from build123d import *

# Parameters (mm, degrees)
SKETCH_1_R          = 19
SKETCH_1_R_2        = 1.45
SKETCH_1_R_3        = 2
EXTRUDE_1_DEPTH     = 12
SKETCH_2_R          = 1.45
SKETCH_2_R_2        = 2
EXTRUDE_2_DEPTH     = 7
SKETCH_3_R          = 1.45
CUT_EXTRUDE_1_DEPTH = 50.298411063
SKETCH_4_R          = 1.45
CUT_EXTRUDE_2_DEPTH = 50.298411063
SKETCH_5_R          = 1.45
CUT_EXTRUDE_3_DEPTH = 8
SKETCH_6_R          = 1.45
CUT_EXTRUDE_4_DEPTH = 46.489925625
CHAMFER_1_SIZE      = 1.55


with BuildPart() as part:
    # 草图1 → 凸台-拉伸1 (new body)
    with BuildSketch(Plane(origin=(0, 0, 0), x_dir=(1, 0, 0), z_dir=(0, 1, 0))):
        with Locations(Location((0, 0, 0), (0, 0, 270))):
            Circle(SKETCH_1_R)
        with Locations(Location((0, 13.5, 0), (0, 0, 270))):
            Circle(SKETCH_1_R_2, mode=Mode.SUBTRACT)
        with Locations(Location((-11.691342951, -6.75, 0), (0, 0, 270))):
            Circle(SKETCH_1_R_2, mode=Mode.SUBTRACT)
        with Locations(Location((11.691342951, -6.75, 0), (0, 0, 270))):
            Circle(SKETCH_1_R_2, mode=Mode.SUBTRACT)
        with Locations(Location((-10.522208656, 6.075, 0), (0, 0, 270))):
            Circle(SKETCH_1_R_3, mode=Mode.SUBTRACT)
        with Locations(Location((0, -12.15, 0), (0, 0, 270))):
            Circle(SKETCH_1_R_3, mode=Mode.SUBTRACT)
        with Locations(Location((10.522208656, 6.075, 0), (0, 0, 270))):
            Circle(SKETCH_1_R_3, mode=Mode.SUBTRACT)
    extrude(amount=EXTRUDE_1_DEPTH)

    # 草图2 → 凸台-拉伸2 (add)
    with BuildSketch(Plane(origin=(0, 12, 0), x_dir=(1, 0, 0), z_dir=(0, 1, 0))):
        Polygon((0, 21.939310229), (-19, 10.969655115), (-19, -10.969655115), (0, -21.939310229), (19, -10.969655115), (19, 10.969655115), align=None)
        with Locations(Location((0, 13.5, 0), (0, 0, 270))):
            Circle(SKETCH_2_R, mode=Mode.SUBTRACT)
        with Locations(Location((-10.522208656, 6.075, 0), (0, 0, 270))):
            Circle(SKETCH_2_R_2, mode=Mode.SUBTRACT)
        with Locations(Location((10.522208656, 6.075, 0), (0, 0, 270))):
            Circle(SKETCH_2_R_2, mode=Mode.SUBTRACT)
        with Locations(Location((-11.691342951, -6.75, 0), (0, 0, 270))):
            Circle(SKETCH_2_R, mode=Mode.SUBTRACT)
        with Locations(Location((0, -12.15, 0), (0, 0, 270))):
            Circle(SKETCH_2_R_2, mode=Mode.SUBTRACT)
        with Locations(Location((11.691342951, -6.75, 0), (0, 0, 270))):
            Circle(SKETCH_2_R, mode=Mode.SUBTRACT)
    extrude(amount=-EXTRUDE_2_DEPTH)

    # 草图3 → 切除-拉伸1 (cut, through all)
    with BuildSketch(Plane(origin=(9.5, 0, 16.454482672), x_dir=(0.8660254037844384, 0, -0.5000000000000004), z_dir=(0.5000000000000004, 0, 0.8660254037844384))):
        with Locations((0, 8.5)):
            Circle(SKETCH_3_R)
    extrude(amount=-CUT_EXTRUDE_1_DEPTH, mode=Mode.SUBTRACT)

    # 草图4 → 切除-拉伸2 (cut, through all)
    with BuildSketch(Plane(origin=(-9.5, 0, 16.454482672), x_dir=(0.8660254037844385, 0, 0.5000000000000004), z_dir=(-0.5000000000000003, 0, 0.8660254037844384))):
        with Locations((0, 8.5)):
            Circle(SKETCH_4_R)
    extrude(amount=-CUT_EXTRUDE_2_DEPTH, mode=Mode.SUBTRACT)

    # 草图5 → 切除-拉伸3 (cut)
    with BuildSketch(Plane.ZY.offset(19)):
        with Locations((0, 8.5)):
            Circle(SKETCH_5_R)
    extrude(amount=-CUT_EXTRUDE_3_DEPTH, mode=Mode.SUBTRACT)

    # 草图6 → 切除-拉伸4 (cut, through all)
    with BuildSketch(Plane(origin=(19, 0, 0), x_dir=(0, 0, -1), z_dir=(1, 0, 0))):
        with Locations(Location((0, 8.5, 0), (0, 0, 180))):
            Circle(SKETCH_6_R)
    extrude(amount=-CUT_EXTRUDE_4_DEPTH, mode=Mode.SUBTRACT)

    # 倒角1
    chamfer_1_edges = [part.edges().sort_by_distance(p)[0] for p in [
        (11.691342951, 12, 5.3),
        (0, 12, -14.95),
        (-11.691342951, 12, 5.3),
    ]]
    chamfer(chamfer_1_edges, length=CHAMFER_1_SIZE)


solid = part.part
Verification items for the finished model (mm, model axes). A direction names the side the tool comes from. Give positions to 0.01 mm unless a question says otherwise; leave off trailing zeros. Write each loop counter-clockwise with the first axis right and the second up, starting at its lowest first coordinate (ties: lowest second). Pieces come first, ordered by that corner, then holes. Notation, with made-up numbers: M 24.5,81 L 30.5,81 A18 cw 30.5,103 Z; hole C 82,-9.5 d6. An arc over 180 degrees is marked long. Write item = value, one per line.
(1) Material ranges on line 1 (Y direction, x = -11, z = 0); line 2 (X direction, y = 8, z = 6.75); line 3 (Z direction, x = -0.5, y = 10.5), recorded low to high.
Found:
line_1 = 0 to 7.05, 9.95 to 12
line_2 = -19 to -13.14, -10.24 to -5.47, -2.33 to 2.33, 5.47 to 10.24, 13.14 to 19
line_3 = -21.65 to -14.91, -12.09 to 10.21, 14.09 to 21.65
(2) Sectioned sample at C-C (y = 6). Record the cut outline in (x, z) (3 decimals).
Found:
outline = M -19,-10.97 L 0,-21.939 L 19,-10.97 L 19,10.97 L 0,21.939 L -19,10.97 Z; hole C -11.691,6.75 d2.9; hole C -10.522,-6.075 d4; hole C 0,12.15 d4; hole C 0,-13.5 d2.9; hole C 10.522,-6.075 d4; hole C 11.691,6.75 d2.9
(3) Sectioned sample at B-B (z = 18). Record the cut outline in (x, y).
Found:
outline = M -6.82,5 L -6.08,5 L -6.08,0 L 6.08,0 L 6.08,5 L 6.82,5 L 6.82,12 L -6.82,12 Z
(4) Access from +Z, -Z, +X, -X, +Y, -Y to the whole of each face (thin tool, end or side, straight path). Record for faces 1 (the face through (-5.94, 8.56, -7.39)), 2 (the face through (17, 5, 10)).
Found:
face_1 = none
face_2 = +Z, +X, -Y
(5) Go/stop test with flat-tipped pins: pin 1 Ø10.5 at (x, z) = (-14, 7) entering from -Y; pin 2 Ø5 at (y, z) = (6, 13.5) entering from +X; pin 3 Ø4 at (x, y) = (-8, 7.5) entering from +Z. Record where each tip stops, or that it passes through.
Found:
pin_1 = 0
pin_2 = 18.95
pin_3 = 18.48
(6) Draft check along X on faces 3 (the face through (-0.555, 5.152, -12.161)), 4 (the face through (0, 5, 20)), 5 (the face through (-19, 10.1, -0.2)), 6 (the face through (5.396, 7.214, 8.008)). Enter one of: released by +X, released by -X, zero draft, split by the parting line, or undercut.
Found:
face_3 = undercut
face_4 = zero draft
face_5 = released by -X
face_6 = undercut
(7) Sectioned sample at A-A (y = 8.5). Give the number of separate pieces and of enclosed holes in the cut face, then the cut area to 3 significant figures.
Found:
separate_pieces = 6
enclosed_holes = 6
area = 884 mm2
